from build123d import *

# Parameters (mm, degrees)
SKETCH1_W           = 50
SKETCH1_H           = 50
BOSS_EXTRUDE1_DEPTH = 10
SKETCH2_W           = 5
SKETCH2_H           = 10
BOSS_EXTRUDE2_DEPTH = 25
SKETCH3_R           = 2
CUT_EXTRUDE1_DEPTH  = 25
SKETCH4_R           = 2
CUT_EXTRUDE2_DEPTH  = 25
FILLET2_R           = 5
FILLET3_R           = 5
FILLET4_R           = 1
FILLET5_R           = 2
FILLET6_R           = 2
SKETCH5_W           = 33
SKETCH5_H           = 33
CUT_EXTRUDE3_DEPTH  = 1
SKETCH6_W           = 15
SKETCH6_H           = 7
CUT_EXTRUDE4_DEPTH  = 16


with BuildPart() as part:
    # Sketch1 → Boss-Extrude1 (new body)
    with BuildSketch(Plane.XY):
        with Locations((25, 25)):
            Rectangle(SKETCH1_W, SKETCH1_H)
    extrude(amount=BOSS_EXTRUDE1_DEPTH)

    # Sketch2 → Boss-Extrude2 (add)
    with BuildSketch(Plane.XZ):
        with Locations((17.5, 5)):
            Rectangle(SKETCH2_W, SKETCH2_H)
        with Locations((32.5, 5)):
            Rectangle(SKETCH2_W, SKETCH2_H)
    extrude(amount=BOSS_EXTRUDE2_DEPTH)

    # Sketch3 → Cut-Extrude1 (cut)
    with BuildSketch(Plane.XY.offset(10)):
        with Locations((43.75, 43.75)):
            Circle(SKETCH3_R)
        with Locations((6.25, 43.75)):
            Circle(SKETCH3_R)
        with Locations((6.25, 6.25)):
            Circle(SKETCH3_R)
        with Locations((43.75, 6.25)):
            Circle(SKETCH3_R)
    extrude(amount=-CUT_EXTRUDE1_DEPTH, mode=Mode.SUBTRACT)

    # Sketch4 → Cut-Extrude2 (cut)
    with BuildSketch(Plane(origin=(35, 0, 0), x_dir=(0, 0, -1), z_dir=(1, 0, 0))):
        with Locations((-5, -10)):
            Circle(SKETCH4_R)
        with Locations((-5, -20)):
            Circle(SKETCH4_R)
    extrude(amount=-CUT_EXTRUDE2_DEPTH, mode=Mode.SUBTRACT)

    # Fillet2
    fillet2_edges = [part.edges().sort_by_distance(p)[0] for p in [
        (32.5, -25, 10),
    ]]
    fillet(fillet2_edges, radius=FILLET2_R)

    # Fillet3
    fillet3_edges = [part.edges().sort_by_distance(p)[0] for p in [
        (17.5, -25, 10),
        (17.5, -25, 0),
        (32.5, -25, 0),
    ]]
    fillet(fillet3_edges, radius=FILLET3_R - 0.0001)  # a hair under: the kernel refuses the full size

    # Fillet4
    fillet4_edges = [part.edges().sort_by_distance(p)[0] for p in [
        (0, 50, 5),
        (50, 50, 5),
        (50, 0, 5),
        (0, 0, 5),
    ]]
    fillet(fillet4_edges, radius=FILLET4_R)

    # Fillet5
    fillet5_edges = [part.edges().sort_by_distance(p)[0] for p in [
        (15, 0, 5),
    ]]
    fillet(fillet5_edges, radius=FILLET5_R)

    # Fillet6
    fillet6_edges = [part.edges().sort_by_distance(p)[0] for p in [
        (35, 0, 5),
    ]]
    fillet(fillet6_edges, radius=FILLET6_R)

    # Sketch5 → Cut-Extrude3 (cut)
    with BuildSketch(Plane.XY.offset(10)):
        with Locations((25, 25)):
            Rectangle(SKETCH5_W, SKETCH5_H)
    extrude(amount=-CUT_EXTRUDE3_DEPTH, mode=Mode.SUBTRACT)

    # Sketch6 → Cut-Extrude4 (cut)
    with BuildSketch(Plane.XY.offset(9)):
        with Locations((20, 12)):
            Rectangle(SKETCH6_W, SKETCH6_H)
    extrude(amount=-CUT_EXTRUDE4_DEPTH, mode=Mode.SUBTRACT)


solid = part.part
Design review of the part built by this model. Coordinates are the model's own, in mm. A direction names the side the tool comes from. Round coordinates to 2 decimals unless told otherwise and drop trailing zeros. Write each loop counter-clockwise with the first axis right and the second up, starting at its lowest first coordinate (ties: lowest second). Pieces come first, ordered by that corner, then holes. Notation, with made-up numbers: (87.5, 0) - (129.5, 0) arc R14 ccw to (129.5, 7) - close; hole circle Ø3 at (3.5, 50). An arc over 180 degrees is marked (long way). Use a Markdown table: item, result. Add a question column.
1. Clearance check with flat-ended pins moving along their axes: pin 1 (5 mm diameter, centred on x = 42.5, z = 3, fed in from -Y); pin 2 (3.5 mm diameter, centred on x = 43.75, y = 6.25, fed in from -Z); pin 3 (3 mm diameter, centred on y = -12.5, z = 6.5, fed in from -X); pin 4 (5 mm diameter, centred on y = -12, z = 7, fed in from +X). State where each tip first meets the part, or that it passes through.
2. We need section B-B (y = 13). State the section outline as (x, z) points.
3. We need section A-A (x = 6.25). State the section outline as (y, z) points, then the cut area to 3 significant figures.
4. Wall thickness on probe 1 along Y at (x, z) = (43.75, 6.75); probe 2 along Y at (x, z) = (21.5, 7.25); probe 3 along X at (y, z) = (-13.5, 4.25): over which ranges is each line inside the solid? List them lowest first.
5. We need section D-D (x = 25). State the section outline as (y, z) points.
6. Mouldability with a two-part tool opening along Y and no side actions: class faces 5 (the face through (35, -13, 5)), 6 (the face through (27.5, 12, 5)), 7 (the face through (35.57, -0.6, 5.07)), 8 (the face through (20, 15.5, 5)) as +Y half, -Y half, draft (parallel to the pull), parting line (faces both ways), or undercut.
7. For faces 1 (the face through (30, -12.3, 4.9)), 2 (the face through (15, -13, 5)), 3 (the face through (25, 25, 9)), 4 (the face through (33, -24, 2)), list the 3-axis set-ups (+Z, -Z, +X, -X, +Y, -Y) from which the entire face can be reached by the end or side of a thin tool; tool diameter is ignored.
Output:
| question | item | result |
|---|---|---|
| 1 | pin 1 | stops at y = 0 |
| 1 | pin 2 | passes through |
| 1 | pin 3 | stops at x = 15 |
| 1 | pin 4 | stops at x = 35 |
| 2 | outline | (0, 0) - (12.5, 0) - (12.5, 9) - (8.5, 9) - (8.5, 10) - (0, 10) - close; (27.5, 0) - (50, 0) - (50, 10) - (41.5, 10) - (41.5, 9) - (27.5, 9) - close |
| 3 | outline | (0, 0) - (4.25, 0) - (4.25, 10) - (0, 10) - close; (8.25, 0) - (41.75, 0) - (41.75, 10) - (8.25, 10) - close; (45.75, 0) - (50, 0) - (50, 10) - (45.75, 10) - close |
| 3 | area | 420 mm2 |
| 4 | probe 1 | y = 0 to 4.25, 8.25 to 41.75, 45.75 to 50 |
| 4 | probe 2 | y = 0 to 8.5, 15.5 to 50 |
| 4 | probe 3 | x = 15 to 20, 30 to 35 |
| 5 | outline | (0, 0) - (8.5, 0) - (8.5, 10) - (0, 10) - close; (15.5, 0) - (50, 0) - (50, 10) - (41.5, 10) - (41.5, 9) - (15.5, 9) - close |
| 6 | face 5 | draft |
| 6 | face 6 | undercut |
| 6 | face 7 | -Y half |
| 6 | face 8 | undercut |
| 7 | face 1 | +Z, -Z, -Y |
| 7 | face 2 | +Z, -Z, -X, -Y |
| 7 | face 3 | +Z |
| 7 | face 4 | -Z, +X, -X, -Y |
